Geometry: final body of the model. Coordinates: model frame, mm. Face numbers are marked on the shaded views. A direction names the side the tool comes from. Give positions to 0.01 mm unless a question says otherwise; leave off trailing zeros. Order: outer loops, then holes, each group sorted by start corner. A loop starts at its lowest first (then second) coordinate and runs counter-clockwise, first axis right, second up. Notation, with made-up numbers: (11.5, -16) -> (46.5, -16) arc R8 cw to (46.5, -10) -> close; hole circle Ø1 at (88.25, -8). An arc over 180 degrees is marked (long way). Answer in a Markdown table with one row per item. Add a question column.
Q1. Cut plane D-D on y = 3.75. Return the cut outline in (x, z), and give its area (3 significant figures).
Q2. Pull-direction query (X, two-part tool) for the marked faces 4, 5 and 6; classes: +X half, -X half, draft (parallel to the pull), parting line (faces both ways), or undercut.
Q3. Cut plane C-C on z = 2. Return the cut outline in (x, y).
Q4. Line query: line 1 along Y through (x, z) = (-15.24, 1); line 2 along Y through (x, z) = (15.24, 0.4); line 3 along X through (y, z) = (0.75, 5.5). Output: solid intervals per line, ascending. Write a range as from..to.
Q5. Cut plane A-A on y = -11.43. Return the cut outline in (x, z), and give its area (3 significant figures).
Q6. Contact query for flat-ended pins moving along their axis: P1, Ø7.5, axis at x = 1.5, y = -8, coming from the +Z side; P2, Ø4.5, axis at x = 4.5, y = 11, coming from the +Z side; P3, Ø1, axis at y = 8, z = 6, coming from the -X side; P4, Ø1.8, axis at x = -15.24, y = 11.43, coming from the +Z side. Output: stop coordinate, or through.
Q7. Set-up query: the marked faces 1, 2 and 3. Return all of +Z, -Z, +X, -X, +Y, -Y with unobstructed straight access to the full face (end or side cutting, diameter ignored); none if empty.
Q8. Cut plane B-B on x = -15.24. Return the cut outline in (y, z), and give its area (3 significant figures).
from build123d import *

# Parameters (mm, degrees)
SKETCH1_W           = 38.1
SKETCH1_H           = 27.94
SKETCH1_R           = 1
BOSS_EXTRUDE1_DEPTH = 1.5
CHAMFER1_SIZE       = 0.5
SKETCH2_W           = 18.758650548
SKETCH2_H           = 15.672811931
SKETCH2_W_2         = 4.719693546
SKETCH2_H_2         = 4.674063521
BOSS_EXTRUDE2_DEPTH = 1
SKETCH3_R           = 3.359281079
BOSS_EXTRUDE3_DEPTH = 6
CHAMFER2_SIZE       = 0.1
FILLET1_R           = 0.5
SKETCH4_W           = 6.703460486
SKETCH4_H           = 15.777656998
BOSS_EXTRUDE4_DEPTH = 8
CHAMFER3_SIZE       = 1


with BuildPart() as part:
    # Sketch1 → Boss-Extrude1 (new body)
    with BuildSketch(Plane.XY):
        Rectangle(SKETCH1_W, SKETCH1_H)
        with Locations((-15.24, 11.43)):
            Circle(SKETCH1_R, mode=Mode.SUBTRACT)
        with Locations((15.24, -11.43)):
            Circle(SKETCH1_R, mode=Mode.SUBTRACT)
    extrude(amount=BOSS_EXTRUDE1_DEPTH)

    # Chamfer1
    chamfer1_edges = [part.edges().sort_by_distance(p)[0] for p in [
        (-19.05, 13.97, 0.75),
        (19.05, 13.97, 0.75),
        (19.05, -13.97, 0.75),
        (-19.05, -13.97, 0.75),
    ]]
    chamfer(chamfer1_edges, length=CHAMFER1_SIZE)

    # Sketch2 → Boss-Extrude2 (add)
    with BuildSketch(Plane.XY.offset(1.5)):
        with Locations((0, -4.770868917)):
            Rectangle(SKETCH2_W, SKETCH2_H)
        with Locations((-8.919164238, 10.689497539)):
            Rectangle(SKETCH2_W_2, SKETCH2_H_2)
    extrude(amount=BOSS_EXTRUDE2_DEPTH)

    # Sketch3 → Boss-Extrude3 (add)
    with BuildSketch(Plane.XY.offset(1.5)):
        with Locations((5.64383642, 9.724451962)):
            Circle(SKETCH3_R)
    extrude(amount=BOSS_EXTRUDE3_DEPTH)

    # Chamfer2
    chamfer2_edges = [part.edges().sort_by_distance(p)[0] for p in [
        (-9.379325274, -4.770868917, 2.5),
        (0, -12.607274882, 2.5),
        (9.379325274, -4.770868917, 2.5),
        (0, 3.065537049, 2.5),
        (-6.559317465, 10.68949754, 2.5),
        (-8.919164238, 13.0265293, 2.5),
        (-11.279011011, 10.68949754, 2.5),
        (-8.919164238, 8.352465779, 2.5),
    ]]
    chamfer(chamfer2_edges, length=CHAMFER2_SIZE)

    # Fillet1
    fillet1_edges = [part.edges().sort_by_distance(p)[0] for p in [
        (2.284555342, 9.724451962, 7.5),
    ]]
    fillet(fillet1_edges, radius=FILLET1_R)

    # Sketch4 → Boss-Extrude4 (add)
    with BuildSketch(Plane.XY.offset(1.5)):
        with Locations((-15.005849453, -0.837932561)):
            Rectangle(SKETCH4_W, SKETCH4_H)
    extrude(amount=BOSS_EXTRUDE4_DEPTH)

    # Chamfer3
    chamfer3_edges = [part.edges().sort_by_distance(p)[0] for p in [
        (-11.65411921, -0.837932561, 9.5),
        (-15.005849453, 7.050895938, 9.5),
        (-18.357579696, -0.837932561, 9.5),
        (-15.005849453, -8.72676106, 9.5),
    ]]
    chamfer(chamfer3_edges, length=CHAMFER3_SIZE)


solid = part.part
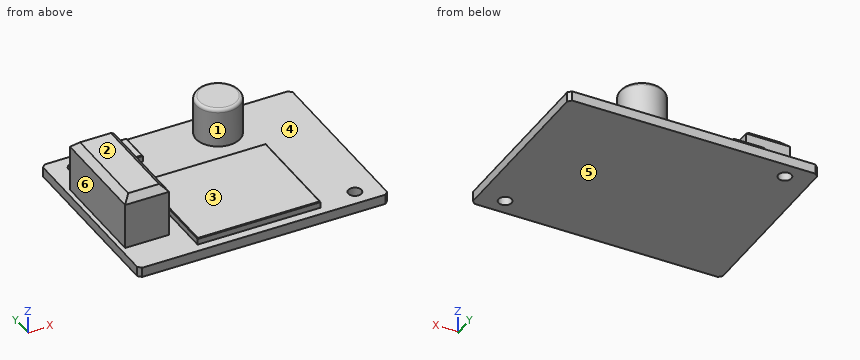
Completed:
| question | item | result |
|---|---|---|
| 1 | outline | (-19.05, 0) -> (19.05, 0) -> (19.05, 1.5) -> (-11.65, 1.5) -> (-11.65, 8.5) -> (-12.65, 9.5) -> (-17.36, 9.5) -> (-18.36, 8.5) -> (-18.36, 1.5) -> (-19.05, 1.5) -> close |
| 1 | area | 110 mm² |
| 2 | face 4 | undercut |
| 2 | face 5 | draft |
| 2 | face 6 | -X half |
| 3 | outline | (-18.36, -8.73) -> (-11.65, -8.73) -> (-11.65, 7.05) -> (-18.36, 7.05) -> close; (-11.28, 8.35) -> (-6.56, 8.35) -> (-6.56, 13.03) -> (-11.28, 13.03) -> close; (-9.38, -12.61) -> (9.38, -12.61) -> (9.38, 3.07) -> (-9.38, 3.07) -> close; circle Ø6.72 at (5.64, 9.72) |
| 4 | line 1 | y = -13.97..10.43, 12.43..13.97 |
| 4 | line 2 | y = -13.97..-12.43, -10.43..13.97 |
| 4 | line 3 | x = -18.36..-11.65 |
| 5 | outline | (-19.05, 0) -> (14.24, 0) -> (14.24, 1.5) -> (9.38, 1.5) -> (9.38, 2.4) -> (9.28, 2.5) -> (-9.28, 2.5) -> (-9.38, 2.4) -> (-9.38, 1.5) -> (-19.05, 1.5) -> close; (16.24, 0) -> (19.05, 0) -> (19.05, 1.5) -> (16.24, 1.5) -> close |
| 5 | area | 72.9 mm² |
| 6 | P1 | stops at z = 2.5 |
| 6 | P2 | stops at z = 7.5 |
| 6 | P3 | stops at x = 2.52 |
| 6 | P4 | passes through |
| 7 | face 1 | +Z |
| 7 | face 2 | +Z, +X, -X, +Y, -Y |
| 7 | face 3 | +Z, +X, -Y |
| 8 | outline | (-13.97, 0) -> (10.43, 0) -> (10.43, 1.5) -> (7.05, 1.5) -> (7.05, 8.5) -> (6.05, 9.5) -> (-7.73, 9.5) -> (-8.73, 8.5) -> (-8.73, 1.5) -> (-13.97, 1.5) -> close; (12.43, 0) -> (13.97, 0) -> (13.97, 1.5) -> (12.43, 1.5) -> close |
| 8 | area | 164 mm² |
